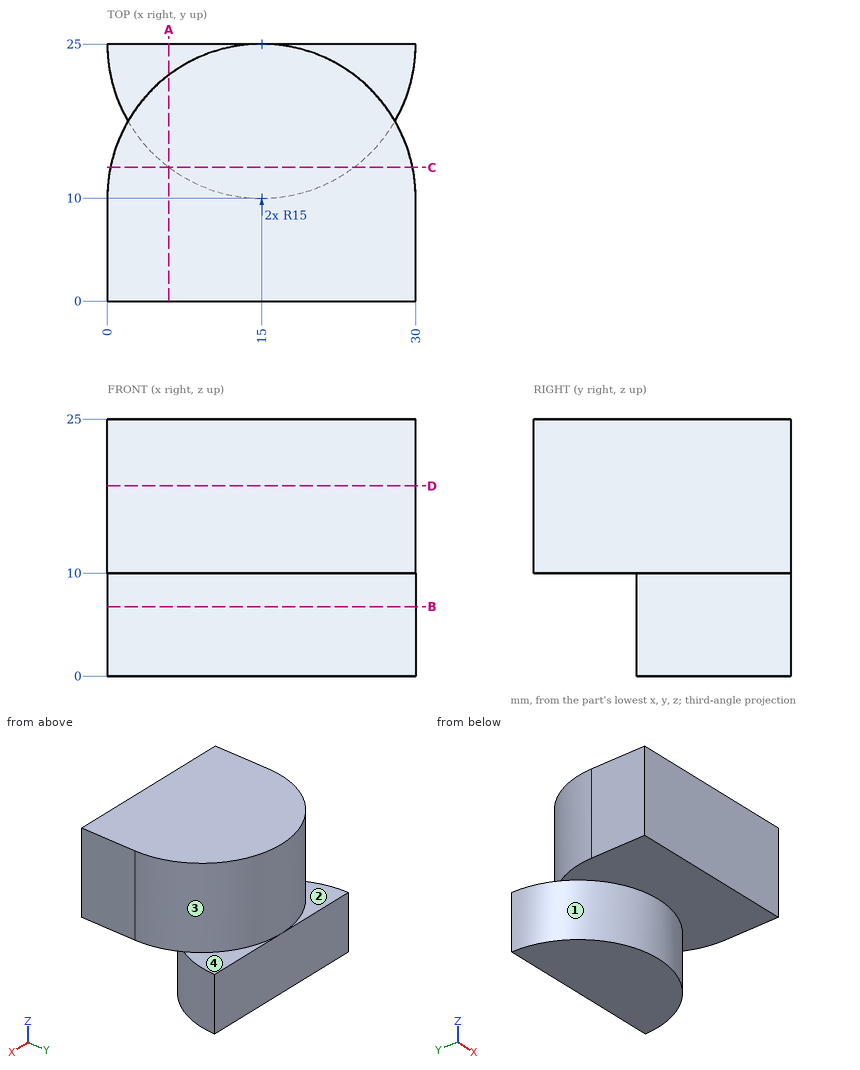
For this review, use the dimensioned drawing (mm, ordinates from the lowest corner) and the shaded views. A direction names the side the tool comes from. Give positions to 0.01 mm unless a question says otherwise; leave off trailing zeros. Order: outer loops, then holes, each group sorted by start corner. A loop starts at its lowest first (then second) coordinate and runs counter-clockwise, first axis right, second up. Notation, with made-up numbers: (10.5, 7) - (25.5, 7) arc R17 cw to (25.5, 32) - close; hole circle Ø8 at (37.25, 42.25). An arc over 180 degrees is marked (long way). Use CSV: the item, a comma, the result in double quotes. Start each with the question number.
Q1. Clearance check with flat-ended pins moving along their axes: pin 1 Ø8 at (y, z) = (15, 13) entering from +X; pin 2 Ø2 at (y, z) = (11.5, 8) entering from +X; pin 3 Ø1.5 at (x, z) = (11, 17.5) entering from +Y. State where each tip first meets the part, or that it passes through.
Q2. We need section D-D, the plane z = 18.5. Write out the cut boundary in (x, y), and give its area (3 significant figures).
Q3. To check wall thickness, follow line 1 along Z through (x, y) = (6.25, 8); line 2 along Z through (x, y) = (2.5, 20.5); line 3 along Y through (x, z) = (15.5, 18). State the ranges of each line that lie inside material, in increasing order. Write a range as [from, to].
Q4. We need section B-B, the plane z = 6.75. Write out the cut boundary in (x, y), and give its area (3 significant figures).
Q5. Tool access review of the marked faces 1, 2, 3 and 4: name each direction out of +Z, -Z, +X, -X, +Y, -Y from which nothing blocks a thin tool from reaching the whole face with its end or side.
Q6. We need section C-C, the plane y = 13. Write out the cut boundary in (x, z).
Q7. We need section A-A, the plane x = 6. Write out the cut boundary in (y, z), and give its area (3 significant figures).
Outcome:
1,pin 1,"stops at x = 29.97"
1,pin 2,"stops at x = 23.29"
1,pin 3,"stops at y = 24.64"
2,outline,"(0, 0) - (30, 0) - (30, 10) arc R15 ccw to (0, 10) - close"
2,area,"653 mm^2"
3,line 1,"z = [10, 25]"
3,line 2,"z = [0, 10]"
3,line 3,"y = [0, 24.99]"
4,outline,"(0, 25) arc R15 ccw to (30, 25) - close"
4,area,"353 mm^2"
5,face 1,"-Z, -Y"
5,face 2,"+Z, -X, +Y"
5,face 3,"+Z, +Y"
5,face 4,"+Z, +X, +Y"
6,outline,"(0.3, 10) - (6, 10) - (6, 0) - (24, 0) - (24, 10) - (29.7, 10) - (29.7, 25) - (0.3, 25) - close"
7,outline,"(0, 10) - (13, 10) - (13, 0) - (25, 0) - (25, 10) - (22, 10) - (22, 25) - (0, 25) - close"
7,area,"450 mm^2"
